Can you work these out from the drawing? Everything is in mm from the part's minimum corner. Coordinates: 2 decimals unless noted, no trailing zeros. Order: outer loops, then holes, each group sorted by start corner. A loop starts at its lowest first (then second) coordinate and runs counter-clockwise, first axis right, second up. Notation, with made-up numbers: (28.5, -19.75) -> (79.5, -19.75) arc R20 ccw to (79.5, 18.25) -> close; hole circle Ø3 at (-22, 59). An arc over 180 degrees is marked (long way). Put each result on its own line as item: value. Start each with the question number.
Q1. If we section it at B-B (y = 1.45): Count the separate pieces of the cut face and the enclosed holes in it, and give its area (3 significant figures).
Q2. If we section it at A-A (z = 65): Please give me the cut outline in (x, y).
Q3. If we section it at C-C (z = 120): Please give me the cut outline in (x, y).
Q4. Will these pins go through, and if not, where does the flat tip stop? pin 1 (1.5 mm diameter, centred on y = 1.5, z = 28.5, fed in from -X); pin 2 (1.5 mm diameter, centred on y = 0.5, z = 104.5, fed in from +X).
Q5. If we section it at D-D (x = 9.5): Please give me the cut outline in (y, z).
Q6. Please list where these lines run through material, in increasing order: line 1 along Z through (x, y) = (22.5, 1.95); line 2 along X through (y, z) = (0.8, 137.5); line 3 along X through (y, z) = (1.8, 2.5).
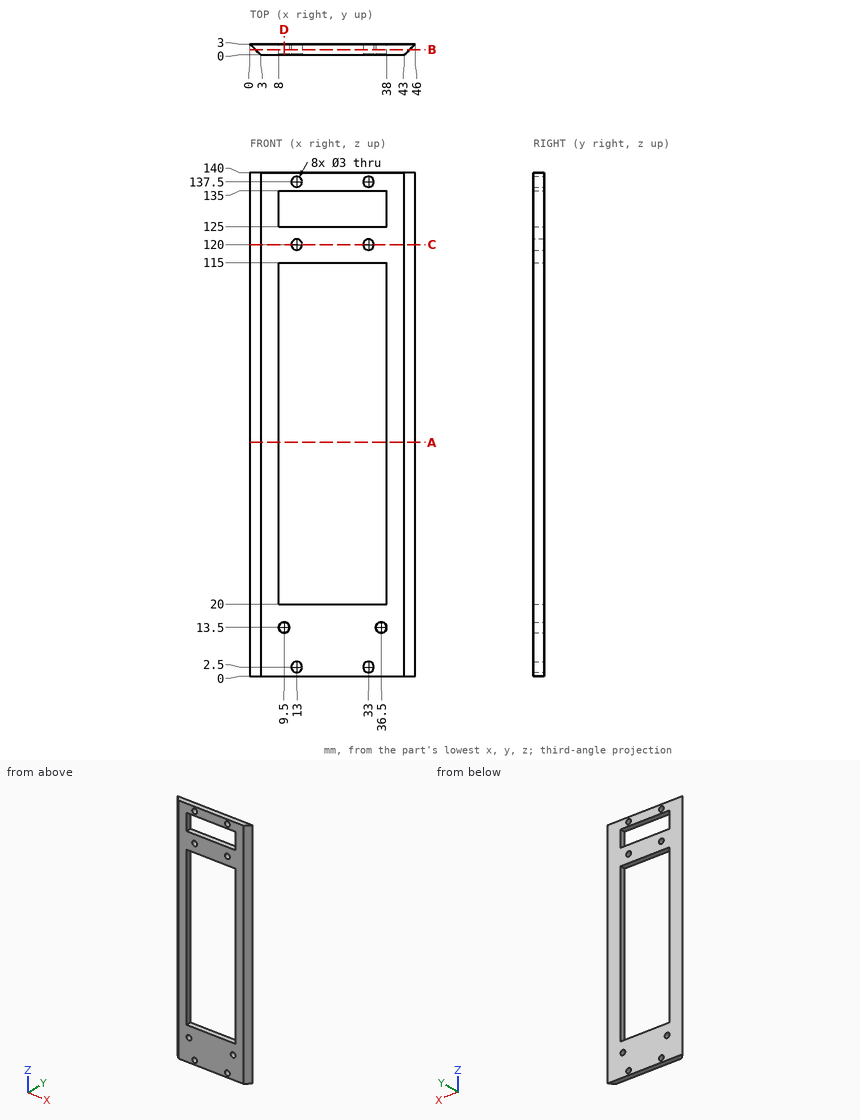
The answers:
1. separate pieces: 1
1. enclosed holes: 10
1. area: 2,800 mm^2
2. outline: (0, 3) -> (3, 0) -> (8, 0) -> (8, 3) -> close; (38, 0) -> (43, 0) -> (46, 3) -> (38, 3) -> close
3. outline: (0, 3) -> (3, 0) -> (11.5, 0) -> (11.5, 3) -> close; (14.5, 0) -> (31.5, 0) -> (31.5, 3) -> (14.5, 3) -> close; (34.5, 0) -> (43, 0) -> (46, 3) -> (34.5, 3) -> close
4. pin 1: x = 0.75
4. pin 2: x = 44.25
5. outline: (0, 0) -> (3, 0) -> (3, 12) -> (0, 12) -> close; (0, 15) -> (3, 15) -> (3, 20) -> (0, 20) -> close; (0, 115) -> (3, 115) -> (3, 125) -> (0, 125) -> close; (0, 135) -> (3, 135) -> (3, 140) -> (0, 140) -> close
6. line 1: 0 to 20, 115 to 125, 135 to 140
6. line 2: 2.2 to 11.5, 14.5 to 31.5, 34.5 to 43.8
6. line 3: 1.2 to 11.5, 14.5 to 31.5, 34.5 to 44.8
